The figure shows three views and two pictorial views of one solid part (mm, origin at its lowest corner). Answer the questions. Coordinates: 2 decimals unless noted, no trailing zeros. Write each loop counter-clockwise with the first axis right and the second up, starting at its lowest first coordinate (ties: lowest second). Pieces come first, ordered by that corner, then holes.
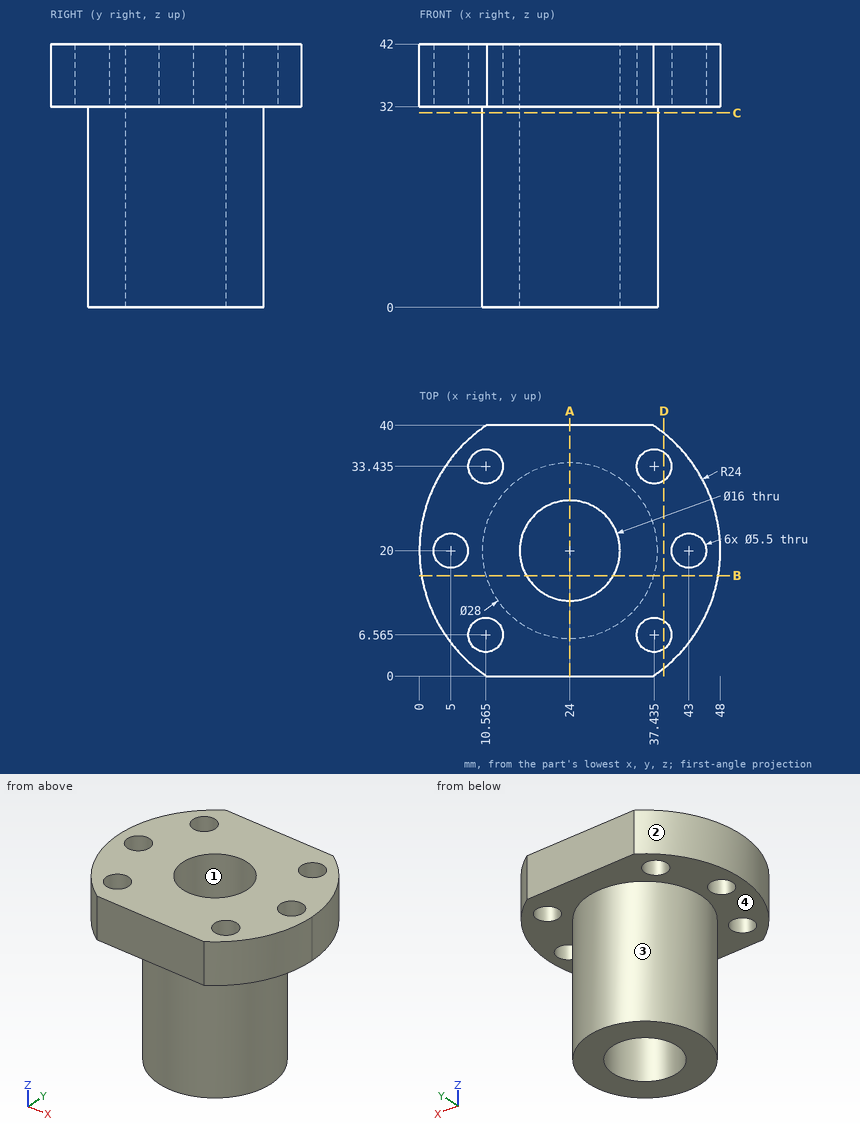
Q1. The part is cut by section D-D, the plane x = 39. Write down the section's boundary in (y, z) (3 decimals), then the cut area to 3 significant figures.
Answers below:
outline: (1.265, 32) - (4.304, 32) - (4.304, 42) - (1.265, 42) - close; (8.826, 32) - (31.174, 32) - (31.174, 42) - (8.826, 42) - close; (35.696, 32) - (38.735, 32) - (38.735, 42) - (35.696, 42) - close
area: 284 mm2
Q2. The part is cut by section A-A, the plane x = 24. Write down the section's boundary in (y, z).
Answers below:
outline: (0, 32) - (6, 32) - (6, 0) - (12, 0) - (12, 42) - (0, 42) - close; (28, 0) - (34, 0) - (34, 32) - (40, 32) - (40, 42) - (28, 42) - close
Q3. The part is cut by section C-C, the plane z = 31. Write down the section's boundary in (x, y), then the cut area to 3 significant figures.
Answers below:
outline: circle Ø28 at (24, 20); hole circle Ø16 at (24, 20)
area: 415 mm2
Q4. Determine the mould class of the marked faces 1, 2, 3 and 4 for opening direction X: released by +X, released by -X, zero draft, split by the parting line, or undercut.
Answers below:
face 1: undercut
face 2: released by -X
face 3: split by the parting line
face 4: zero draft
Q5. The part is cut by section B-B, the plane y = 16. Write down the section's boundary in (x, z).
Answers below:
outline: (0.34, 32) - (10.58, 32) - (10.58, 0) - (17.07, 0) - (17.07, 42) - (0.34, 42) - close; (30.93, 0) - (37.42, 0) - (37.42, 32) - (47.66, 32) - (47.66, 42) - (30.93, 42) - close
Q6. Find the intervals of material crossed by probe 1 along Y at (x, z) = (24, 20); probe 2 along X at (y, z) = (20.5, 31.5); probe 3 along X at (y, z) = (26.5, 27), in increasing order.
Answers below:
probe 1: y = 6 to 12, 28 to 34
probe 2: x = 10.01 to 16.02, 31.98 to 37.99
probe 3: x = 11.6 to 19.34, 28.66 to 36.4
Q7. Given pin 1 (6 mm diameter, centred on x = 17.5, z = 10.5, fed in from -Y); pin 2 (5 mm diameter, centred on x = 21, z = 8.5, fed in from +Y); pin 3 (6.5 mm diameter, centred on x = 37.44, y = 6.56, fed in from -Z), each flat-ended and moving along its own axis, determine where each tip first touches the part or whether it passes through.
Answers below:
pin 1: stops at y = 6.44
pin 2: stops at y = 33.99
pin 3: stops at z = 32
